Geometry check sheet. Reference: the model listing, model coordinates, mm. Give positions to 0.01 mm unless a question says otherwise; leave off trailing zeros. Order: outer loops, then holes, each group sorted by start corner. A loop starts at its lowest first (then second) coordinate and runs counter-clockwise, first axis right, second up. Notation, with made-up numbers: M 81,-36 L 115,-36 A38 cw 115,2 Z; hole C 72,73.25 d11. An arc over 180 degrees is marked long. Answer as CSV lines item,"result".
from build123d import *

# Parameters (mm, degrees)
SKETCH_1_W          = 25
SKETCH_1_H          = 200
SKETCH_1_R          = 2
SKETCH_1_R_2        = 1.5
SKETCH_1_R_3        = 2.05
EXTRUDE_1_DEPTH     = 3
FILLET_1_R          = 8
CUT_EXTRUDE_1_REACH = 203.579
SKETCH_3_R          = 1.55


with BuildPart() as part:
    # 草图1 → 凸台-拉伸1 (new body)
    with BuildSketch(Plane.XY):
        with Locations((12.5, 100)):
            Rectangle(SKETCH_1_W, SKETCH_1_H)
        with Locations((7.5, 6)):
            Circle(SKETCH_1_R, mode=Mode.SUBTRACT)
        with Locations(Location((17.5, 6, 0), (0, 0, 180))):
            Circle(SKETCH_1_R, mode=Mode.SUBTRACT)
        with Locations((12.5, 19.055282456)):
            Circle(SKETCH_1_R, mode=Mode.SUBTRACT)
        with Locations((5.782485579, 178.282485579)):
            Circle(SKETCH_1_R_2, mode=Mode.SUBTRACT)
        with Locations((5.782485579, 191.717514421)):
            Circle(SKETCH_1_R_2, mode=Mode.SUBTRACT)
        with Locations((19.217514421, 191.717514421)):
            Circle(SKETCH_1_R_2, mode=Mode.SUBTRACT)
        with Locations((19.217514421, 178.282485579)):
            Circle(SKETCH_1_R_2, mode=Mode.SUBTRACT)
        with Locations((12.5, 50.562827646)):
            Circle(SKETCH_1_R_3, mode=Mode.SUBTRACT)
    extrude(amount=EXTRUDE_1_DEPTH)

    # 圆角1
    fillet_1_edges = [part.edges().sort_by_distance(p)[0] for p in [
        (0, 200, 1.5),
        (25, 200, 1.5),
        (25, 0, 1.5),
        (0, 0, 1.5),
    ]]
    fillet(fillet_1_edges, radius=FILLET_1_R)

    # 草图3 → 切除-拉伸1 (cut, up to next)
    with BuildSketch(Plane.XY.offset(3), mode=Mode.PRIVATE) as cut_extrude_1_sk1:
        with Locations((21.5, 50.562827646)):
            Circle(SKETCH_3_R)
    cut_extrude_1_tool1 = extrude(cut_extrude_1_sk1.sketch, amount=-CUT_EXTRUDE_1_REACH, mode=Mode.PRIVATE) & part.part
    # 草图3 → 切除-拉伸1 (cut, up to next)
    with BuildSketch(Plane.XY.offset(3), mode=Mode.PRIVATE) as cut_extrude_1_sk2:
        with Locations((3.5, 50.562827646)):
            Circle(SKETCH_3_R)
    cut_extrude_1_tool2 = extrude(cut_extrude_1_sk2.sketch, amount=-CUT_EXTRUDE_1_REACH, mode=Mode.PRIVATE) & part.part
    add(cut_extrude_1_tool1.solids().sort_by_distance((21.5, 50.562828, 3))[0], mode=Mode.SUBTRACT)
    add(cut_extrude_1_tool2.solids().sort_by_distance((3.5, 50.562828, 3))[0], mode=Mode.SUBTRACT)


solid = part.part
(1) Gauge pin test, flat end, axial feed: P1, Ø3, axis at x = 21.5, y = 50.56, coming from the -Z side. Record the tip position at first contact, or that the pin passes through.
The answers:
P1,"passes through"
(2) Draft check along Y on faces 1 (the face through (12, 101, 0)), 2 (the face through (22.594, 2.281, 1.521)), 3 (the face through (21.3, 52.1, 1.5)). Enter one of: +Y half, -Y half, draft (parallel to the pull), parting line (faces both ways), or undercut.
The answers:
face 1,"draft"
face 2,"-Y half"
face 3,"undercut"
(3) Section check A-A on x = 12.5. Enter the section's corners in (y, z), then the cut area to 3 significant figures.
The answers:
outline,"M 0,0 L 17.06,0 L 17.06,3 L 0,3 Z; M 21.06,0 L 48.51,0 L 48.51,3 L 21.06,3 Z; M 52.61,0 L 200,0 L 200,3 L 52.61,3 Z"
area,"576 mm2"
(4) Material ranges on line 1 (Y direction, x = 12.5, z = 1.5); line 2 (X direction, y = 179, z = 0.45); line 3 (Y direction, x = 7.5, z = 2.2), recorded low to high.
The answers:
line 1,"y = 0 to 17.06, 21.06 to 48.51, 52.61 to 200"
line 2,"x = 0 to 4.47, 7.1 to 17.9, 20.53 to 25"
line 3,"y = 0.02 to 4, 8 to 199.98"
(5) Section check B-B on z = 0.65. State how many separate pieces and enclosed holes the cut face has, then the cut area to 3 significant figures.
The answers:
separate pieces,"1"
enclosed holes,"10"
area,"4,850 mm2"
